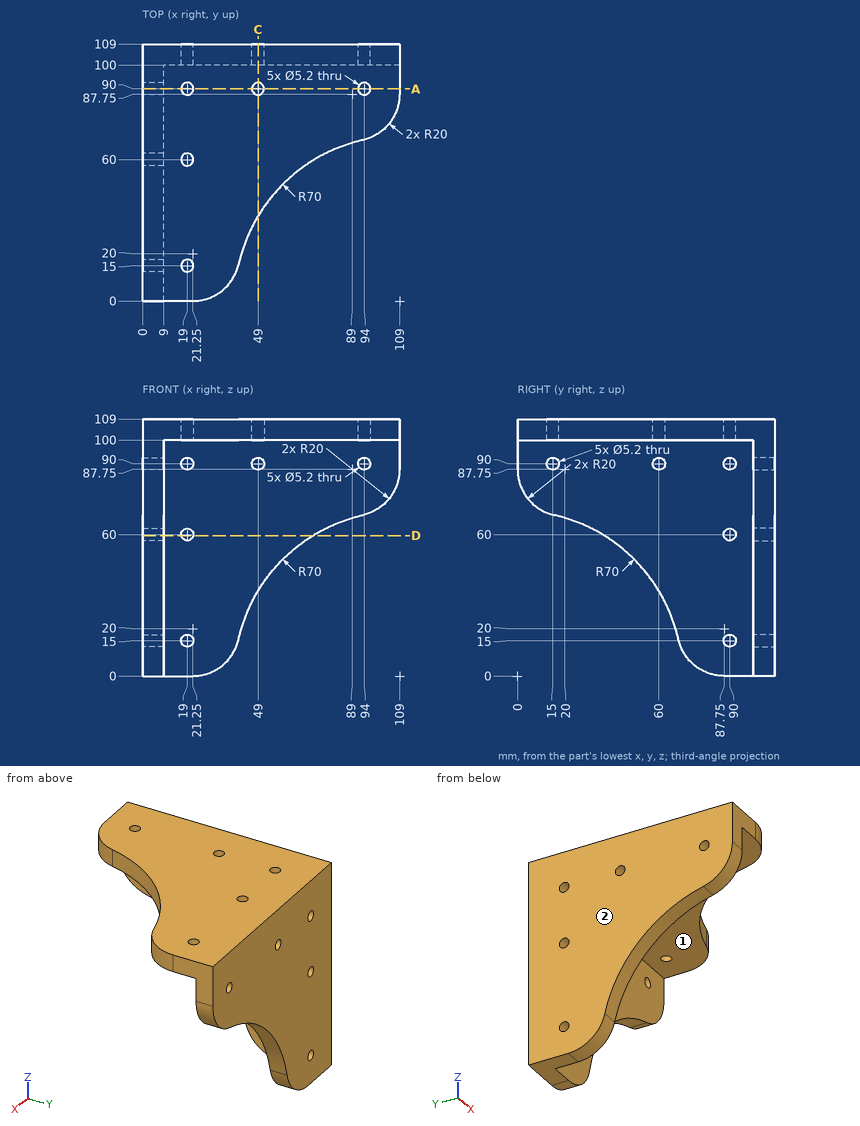
Input: dimensioned drawing with shaded views. Units: mm. Origin: part minimum x, y, z. A direction names the side the tool comes from. Round coordinates to 2 decimals unless told otherwise and drop trailing zeros. Order: outer loops, then holes, each group sorted by start corner. A loop starts at its lowest first (then second) coordinate and runs counter-clockwise, first axis right, second up. Notation, with made-up numbers: (28.5, -20.75) -> (37.5, -20.75) arc R32 ccw to (37.5, 16.25) -> close; hole circle Ø6 at (81, -21.5). An arc over 180 degrees is marked (long way). One line per item, written item: value. Start each with the question number.
Q1. Material intervals for probe 1 along Y at (x, z) = (19, 105.25); probe 2 along X at (y, z) = (105.75, 90); probe 3 along X at (y, z) = (91, 70), sorted ascending.
Q2. Section query A-A (y = 90). Give the number of separate pieces and of enclosed holes in the cut face, plus the area to 3 significant figures.
Q3. Access query for the marked faces 1 and 2. Directions: +Z, -Z, +X, -X, +Y, -Y. A direction counts if a zero-diameter tool reaches every point of the face in a straight line with its end or side. Return the directions, or none.
Q4. Section query D-D (z = 59.5). Return the cut outline in (x, y) (1 decimal), plus the area to 3 significant figures.
Q5. Section query C-C (x = 49). Return the cut outline in (y, z) (1 decimal).
Q6. Pin query (flat end, axial travel): pin 1 (3 mm diameter, centred on y = 15, z = 90, fed in from +X); pin 2 (1 mm diameter, centred on y = 92.5, z = 63.5, fed in from +X); pin 3 (6 mm diameter, centred on x = 19, z = 90, fed in from -Y). Return the tip coordinate at first contact, or that it passes through.
Findings below:
1. probe 1: 0 to 12.4, 17.6 to 57.4, 62.6 to 87.4, 92.6 to 109
1. probe 2: 0 to 16.4, 21.6 to 46.4, 51.6 to 91.4, 96.6 to 109
1. probe 3: 0 to 9
2. separate pieces: 7
2. enclosed holes: 0
2. area: 1,600 mm²
3. face 1: -Z, +X, -Y
3. face 2: +Z, -Z, -X, +Y, -Y
4. outline: (0, 36.9) -> (9, 36.9) -> (9, 87.4) -> (0, 87.4) -> close; (0, 92.6) -> (9, 92.6) -> (9, 100) -> (16.4, 100) -> (16.4, 109) -> (0, 109) -> close; (21.6, 100) -> (72.1, 100) -> (72.1, 109) -> (21.6, 109) -> close
4. area: 1,130 mm²
5. outline: (36.1, 100) -> (87.4, 100) -> (87.4, 109) -> (36.1, 109) -> close; (92.6, 100) -> (100, 100) -> (100, 92.6) -> (109, 92.6) -> (109, 109) -> (92.6, 109) -> close; (100, 36.1) -> (109, 36.1) -> (109, 87.4) -> (100, 87.4) -> close
6. pin 1: through
6. pin 2: x = 9
6. pin 3: y = 100
